Read the model definition and answer for the solid it produces. Units are mm, in the model's axes. Face numbers are marked on the shaded views. A direction names the side the tool comes from. Give positions to 0.01 mm unless a question says otherwise; leave off trailing zeros. Write each loop counter-clockwise with the first axis right and the second up, starting at its lowest first coordinate (ties: lowest second). Pieces come first, ordered by that corner, then holes.
```python
from build123d import *

# Parameters (mm, degrees)
SKETCH_1_W          = 15
SKETCH_1_H          = 50
EXTRUDE_1_DEPTH     = 5
EXTRUDE_2_DEPTH     = 5
FILLET_1_R          = 4
FILLET_3_R          = 2
SKETCH_5_R          = 1.6
CUT_EXTRUDE_1_DEPTH = 5
SKETCH_7_R          = 1.5
EXTRUDE_3_DEPTH     = 5
CHAMFER_1_SIZE      = 2.5
FILLET_8_R          = 3
EXTRUDE_4_DEPTH     = 3
FILLET_9_R          = 2


with BuildPart() as part:
    # 草图1 → 凸台-拉伸1 (new body)
    with BuildSketch(Plane(origin=(0, 0, 0), x_dir=(1, 0, 0), z_dir=(0, 1, 0))):
        Rectangle(SKETCH_1_W, SKETCH_1_H)
        Polygon((13.5, -25), (7.5, -25), (7.5, 25), align=None)
    extrude(amount=EXTRUDE_1_DEPTH)

    # 草图4 → 凸台-拉伸2 (add)
    with BuildSketch(Plane.ZY.offset(7.5)):
        Polygon((-25, 6), (-25, 5), (25, 5), (25, 12), (15, 12), (15, 7), align=None)
    extrude(amount=-EXTRUDE_2_DEPTH)

    # 圆角1
    fillet_1_edges = [part.edges().sort_by_distance(p)[0] for p in [
        (-5, 6, -25),
    ]]
    fillet(fillet_1_edges, radius=FILLET_1_R)

    # 圆角3
    fillet_3_edges = [part.edges().sort_by_distance(p)[0] for p in [
        (-5, 12, 15),
    ]]
    fillet(fillet_3_edges, radius=FILLET_3_R)

    # 草图5 → 切除-拉伸1 (cut)
    with BuildSketch(Plane(origin=(0, 5, 0), x_dir=(1, 0, 0), z_dir=(0, 1, 0))):
        with Locations(Location((2.5, 20, 0), (0, 0, 270))):
            Circle(SKETCH_5_R)
        with Locations(Location((2.5, 0, 0), (0, 0, 270))):
            Circle(SKETCH_5_R)
        with Locations(Location((2.5, -20, 0), (0, 0, 270))):
            Circle(SKETCH_5_R)
    extrude(amount=-CUT_EXTRUDE_1_DEPTH, mode=Mode.SUBTRACT)

    # 草图7 → 凸台-拉伸3 (add)
    with BuildSketch(Plane.XY.offset(25)):
        Polygon((13.5, 0), (13.5, 5), (-2.5, 5), (-2.5, 12), (-7.5, 12), (-7.5, 0), (-7.5, -12), (13.5, -12), align=None)
        with Locations((-1.5, -7)):
            Circle(SKETCH_7_R, mode=Mode.SUBTRACT)
        with Locations((7.5, -7)):
            Circle(SKETCH_7_R, mode=Mode.SUBTRACT)
    extrude(amount=EXTRUDE_3_DEPTH)

    # 倒角1
    chamfer_1_edges = [part.edges().sort_by_distance(p)[0] for p in [
        (3, 0, 25),
    ]]
    chamfer(chamfer_1_edges, length=CHAMFER_1_SIZE)

    # 圆角8
    fillet_8_edges = [part.edges().sort_by_distance(p)[0] for p in [
        (-5, 12, 30),
    ]]
    fillet(fillet_8_edges, radius=FILLET_8_R)

    # 草图8 → 凸台-拉伸4 (add)
    with BuildSketch(Plane.ZY.offset(7.5)):
        Polygon((25, -12), (25, -2.5), (22.5, 0), (-7.5, 0), align=None)
    extrude(amount=-EXTRUDE_4_DEPTH)

    # 圆角9
    fillet_9_edges = [part.edges().sort_by_distance(p)[0] for p in [
        (13.5, -12, 27.5),
        (-7.5, -12, 27.5),
    ]]
    fillet(fillet_9_edges, radius=FILLET_9_R)


solid = part.part
```
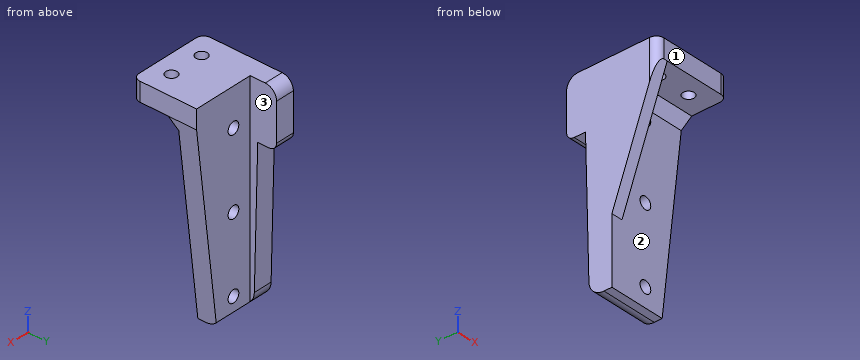
Item 1: Which of the six approach directions +Z, -Z, +X, -X, +Y, -Y give full straight-line access (tool end or side, diameter ignored) to the marked faces 1, 2 and 3?
Result set:
face 1: +Z, -Z, +X, -X, -Y
face 2: -Z, +X, -Y
face 3: +Z, -Z, +X, +Y
Item 2: Section B-B (y = 1.25) is taken. Write down the section's boundary in (x, z), and give its area (3 significant figures).
Result set:
outline: (-7.5, -25) - (7.5, -25) - (13.5, 25) - (13.5, 30) - (-7.5, 30) - close; hole circle Ø3.2 at (2.5, -20); hole circle Ø3.2 at (2.5, 0); hole circle Ø3.2 at (2.5, 20)
area: 981 mm2
Item 3: Find the intervals of material crossed by line 1 along Y through (x, z) = (-1.5, 26.15); line 2 along X through (y, z) = (-5.75, 24); line 3 along X through (y, z) = (1.75, 20), in increasing order.
Result set:
line 1: y = -12 to -8.5, -5.5 to 5
line 2: x = -7.5 to -4.5
line 3: x = -7.5 to 0.9, 4.1 to 12.9
Item 4: Section D-D (x = 10.5) is taken. Write down the section's boundary in (y, z).
Result set:
outline: (-12, 25) - (-2.5, 25) - (0, 22.5) - (0, 0) - (5, 0) - (5, 30) - (-12, 30) - close
Item 5: Each of these flat-tipped pins is pushed along its axis until it touches: pin 1 Ø3 at (x, z) = (2.5, 20) entering from +Y; pin 2 Ø1.5 at (x, y) = (-5.5, 8.5) entering from -Z; pin 3 Ø10.5 at (x, z) = (1.5, 1) entering from -Y; pin 4 Ø9.5 at (y, z) = (-5.5, 7) entering from +X. Where does it stop, or does it pass through?
Result set:
pin 1: passes through
pin 2: stops at z = 15
pin 3: stops at y = 0
pin 4: stops at x = -4.5
Item 6: Section A-A (x = -1.5) is taken. Write down the section's boundary in (y, z), and give its area (3 significant figures).
Result set:
outline: (-12, 25) - (-8.5, 25) - (-8.5, 30) - (-12, 30) - close; (-5.5, 25) - (-2.5, 25) - (0, 22.5) - (0, -25) - (2.1, -25) arc R4 ccw to (5, -23.75) - (5, 30) - (-5.5, 30) - close
area: 322 mm2
Item 7: Section C-C (z = 0) is taken. Write down the section's boundary in (x, y) (3 decimals).
Result set:
outline: (-7.5, -2.769) - (-4.5, -2.769) - (-4.5, 0) - (0.9, 0) - (0.9, 5) - (-2.5, 5) - (-2.5, 6.625) - (-7.5, 6.625) - close; (4.1, 0) - (10.5, 0) - (10.5, 5) - (4.1, 5) - close
